Read the model definition and answer for the solid it produces. Units are mm, in the model's axes. Face numbers are marked on the shaded views. A direction names the side the tool comes from. Give positions to 0.01 mm unless a question says otherwise; leave off trailing zeros. Order: outer loops, then holes, each group sorted by start corner. A loop starts at its lowest first (then second) coordinate and runs counter-clockwise, first axis right, second up. Notation, with made-up numbers: (-32, 57) - (4, 57) arc R18 cw to (4, 89) - close; hole circle Ø9 at (88.25, -32.75). An arc over 180 degrees is marked (long way). Write each question's results on one line, items separated by ' | '. Start each with the question number.
Q1. Find the intervals of material crossed by line 1 along Y through (x, z) = (32.5, 6.5); line 2 along Y through (x, z) = (12, 5); line 3 along Z through (x, y) = (5, 40.5), in increasing order. Write a range as from..to.
Q2. Find section D-D on z = 17.75. Give the vertices of the cut face in (x, y).
Q3. A tool of negligible diameter and unlimited length cuts with its end or side. For the marked faces 1, 2 and 3, from which of +Z, -Z, +X, -X, +Y, -Y can it reach the whole face along a straight path? Write none if from no direction.
Q4. Find section B-B on z = 10. Give the vertices of the cut face in (x, y), and give its area (3 significant figures).
Q5. Find section C-C on x = 20.5. Give the vertices of the cut face in (y, z).
Q6. Flat-ended cylindrical pins translate along their axes: P1, Ø1.5, axis at x = 15, z = 8, coming from the +Y side; P2, Ø10.5, axis at x = 12.5, z = 7, coming from the -Y side. Find the tip coordinate at first contact, or state that the pin passes through.
Q7. Find section A-A on x = 10. Give the vertices of the cut face in (y, z).
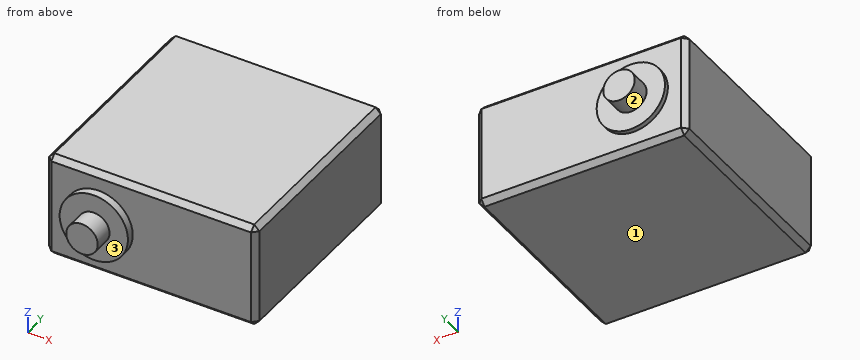
Autodesk Inventor part; units mm, degrees
ref_plane "YZ Plane" through (0, 0, 0) normal (1, 0, 0) x (0, 1, 0)
ref_plane "XZ Plane" through (0, 0, 0) normal (0, 1, 0) x (-1, 0, 0)
ref_plane "XY Plane" through (0, 0, 0) normal (0, 0, 1) x (1, 0, 0)
sketch "Sketch1" plane through (0, 0, 0) normal (0, 0, 1) x (1, 0, 0)
  line L0 (0, 0) -> (40, 0)
  line L1 (40, 0) -> (40, 40)
  line L2 (40, 40) -> (0, 40)
  line L3 (0, 40) -> (0, 0)
  dimension "d0" = 40
  dimension "d1" = 40
extrude "Extrusion1" add sketch "Sketch1" along normal blind 20
chamfer "Chamfer1" distance 1 angle 45 12 edges at (20, 40, 20) (20, 40, 0) (40, 40, 10) (40, 20, 20) (40, 20, 0) (40, 0, 10) (20, 0, 20) (0, 20, 20) (0, 40, 10) (0, 20, 0) (0, 0, 10) (20, 0, 0)
sketch "Sketch2" plane through (1, 40, 1) normal (0, 1, 0) x (1, 0, 0)
  line L0 (-1, -18) -> (-1, 0)
  line L1 (-1, -9) -> (9, -9)
  circle A0 centre (9, -9) radius 3
  point P0 (-1, 1)
  dimension "d7" = 10
  dimension "d8" = 6
extrude "Extrusion2" add sketch "Sketch2" along normal blind 4.6
sketch "Sketch3" plane through (1, 40, 1) normal (0, 1, 0) x (1, 0, 0)
  circle A0 centre (9, -9) radius 3
  circle A1 centre (9, -9) radius 6.5
  point P0 (-1, 1)
  dimension "d11" = 13
extrude "Extrusion3" add sketch "Sketch3" along normal blind 0.9
sketch "Sketch5" plane through (1, 0, 19) normal (0, -1, 0) x (1, 0, 0)
  line L0 (-1, 0) -> (-1, -18)
  line L1 (-1, -9) -> (9, -9)
  circle A0 centre (9, -9) radius 3
  point P0 (-1, -19)
  dimension "d14" = 10
extrude "Extrusion4" add sketch "Sketch5" along normal blind 5.2
sketch "Sketch6" plane through (1, 0, 19) normal (0, -1, 0) x (1, 0, 0)
  circle A0 centre (9, -9) radius 3
  circle A1 centre (9, -9) radius 6.5
  point P0 (-1, -19)
  dimension "d17" = 13
extrude "Extrusion5" add sketch "Sketch6" along normal blind 1.5 contours A0 | A1
properties part number "DualServo"
Working result:
1) line 1: 0..40 | line 2: -1.5..40.9 | line 3: 5.85..14.15
2) outline: (0, 1) - (1, 0) - (39, 0) - (40, 1) - (40, 39) - (39, 40) - (1, 40) - (0, 39) - close
3) face 1: -Z, +X, -X, +Y, -Y | face 2: +Y | face 3: -Y
4) outline: (0, 1) - (1, 0) - (3.5, 0) - (3.5, -1.5) - (7, -1.5) - (7, -5.2) - (13, -5.2) - (13, -1.5) - (16.5, -1.5) - (16.5, 0) - (39, 0) - (40, 1) - (40, 39) - (39, 40) - (16.5, 40) - (16.5, 40.9) - (13, 40.9) - (13, 44.6) - (7, 44.6) - (7, 40.9) - (3.5, 40.9) - (3.5, 40) - (1, 40) - (0, 39) - close | area: 1,670 mm²
5) outline: (0, 1) - (1, 0) - (39, 0) - (40, 1) - (40, 19) - (39, 20) - (1, 20) - (0, 19) - close
6) P1: y = 40.9 | P2: y = -5.2
7) outline: (-5.2, 7) - (-1.5, 7) - (-1.5, 3.5) - (0, 3.5) - (0, 1) - (1, 0) - (39, 0) - (40, 1) - (40, 3.5) - (40.9, 3.5) - (40.9, 7) - (44.6, 7) - (44.6, 13) - (40.9, 13) - (40.9, 16.5) - (40, 16.5) - (40, 19) - (39, 20) - (1, 20) - (0, 19) - (0, 16.5) - (-1.5, 16.5) - (-1.5, 13) - (-5.2, 13) - close
